```python
from build123d import *

# Parameters (mm, degrees)
F0_W     = 25.4
F0_H     = 25.4
F0_W_2   = 19.05
F0_H_2   = 19.05
F1_DEPTH = 218.28125
F2_R     = 2.38125
F3_DEPTH = 25.401
F4_R     = 2.38125
F5_DEPTH = 25.401


with BuildPart() as f1:
    # F0 (on Front) → F1 (new body, symmetric)
    with BuildSketch(Plane.XZ):
        Rectangle(F0_W, F0_H)
        Rectangle(F0_W_2, F0_H_2, mode=Mode.SUBTRACT)
    extrude(amount=F1_DEPTH, both=True)

    # F2 (on face) → F3 (cut, through all)
    with BuildSketch(Plane.XY.offset(12.7)):
        with Locations((0, -205.58125)):
            Circle(F2_R)
        with Locations((0, -180.18125)):
            Circle(F2_R)
    extrude(amount=-F3_DEPTH, mode=Mode.SUBTRACT)

    # F4 (on face) → F5 (cut, through all)
    with BuildSketch(Plane.YZ.offset(12.7)):
        with Locations((192.88125, 0)):
            Circle(F4_R)
        with Locations((116.68125, 0)):
            Circle(F4_R)
    extrude(amount=-F5_DEPTH, mode=Mode.SUBTRACT)


solid = f1.part
```
Here's how the part is built. I have some questions about the finished solid (model axes, mm). A direction names the side the tool comes from. Give positions to 0.01 mm unless a question says otherwise; leave off trailing zeros. Order: outer loops, then holes, each group sorted by start corner. A loop starts at its lowest first (then second) coordinate and runs counter-clockwise, first axis right, second up. Notation, with made-up numbers: M 7.5,19.5 L 38.5,19.5 A38 cw 38.5,58.5 Z; hole C -14.5,-26 d9. An arc over 180 degrees is marked long. Use a Markdown table: item, result. Add a question column.
1. If we mould it in two halves opening along X, with no side actions, what happens to faces 1 (the flat face through (-9.525, -3, 0)), 2 (the flat face through (12.7, -3, 0)), 3 (the flat face through (11, -218.281, 0))? For each: +X half, -X half, draft (parallel to the pull), parting line (faces both ways), or undercut.
2. Suppose I cut it at A-A (y = 110.5). List the corners of the cut face in (x, z) for me (3 decimals), and give its area (3 significant figures).
3. For pin 1 Ø4 at (y, z) = (116.68, 0) entering from -X; pin 2 Ø5.5 at (x, y) = (0, -205.58) entering from -Z, each with a flat end and sliding along its axis, tell me the tip position at first contact or that it passes through.
4. On a 3-axis mill with a long thin cutter (end or side, diameter ignored), from which of +Z, -Z, +X, -X, +Y, -Y can I reach the whole of each face in a straight line? I mean faces 4 (the flat face through (0, -3, -12.7)), 5 (the flat face through (0, -3, -9.525)). Say none if no direction works.
5. I need wall thicknesses on probe 1 along Y at (x, z) = (0, -10.9); probe 2 along Z at (x, y) = (-4.75, 43) (3 decimals). Which ranges of each line are inside material? Lowest first, please. Write a range as from..to.
Results list:
| question | item | result |
|---|---|---|
| 1 | face 1 | undercut |
| 1 | face 2 | +X half |
| 1 | face 3 | draft |
| 2 | outline | M -12.7,-12.7 L 12.7,-12.7 L 12.7,12.7 L -12.7,12.7 Z; hole M -9.525,-9.525 L 9.525,-9.525 L 9.525,9.525 L -9.525,9.525 Z |
| 2 | area | 282 mm² |
| 3 | pin 1 | passes through |
| 3 | pin 2 | stops at z = -12.7 |
| 4 | face 4 | -Z, +X, -X, +Y, -Y |
| 4 | face 5 | +Y, -Y |
| 5 | probe 1 | y = -218.28..-207.96, -203.2..-182.56, -177.8..218.28 |
| 5 | probe 2 | z = -12.7..-9.525, 9.525..12.7 |
